Verification items for the finished model (mm, model axes). A direction names the side the tool comes from. Round coordinates to 2 decimals unless told otherwise and drop trailing zeros. Order: outer loops, then holes, each group sorted by start corner. A loop starts at its lowest first (then second) coordinate and runs counter-clockwise, first axis right, second up. Notation, with made-up numbers: M 72,64 L 121,64 A23 ccw 121,93 Z; hole C -34.5,-24 d3. An arc over 180 degrees is marked long. Return JSON: item names as keys, results as strings. Group by question number.
from build123d import *

# Parameters (mm, degrees)
F0_R     = 1
F0_R_2   = 3
F1_DEPTH = 2


with BuildPart() as f1:
    # F0 (on Top) → F1 (new body)
    with BuildSketch(Plane.XY):
        with BuildLine():
            Line((6.85, -35.27), (6.85, -9.66954))
            ThreePointArc((6.85, -9.66954), (10.262401, -5.925), (11.799067, -1.097504))
            Line((11.799067, -1.097504), (33.969716, 11.702726))
            Line((33.969716, 11.702726), (27.119716, 23.567274))
            Line((27.119716, 23.567274), (4.949067, 10.767044))
            ThreePointArc((4.949067, 10.767044), (0, 11.85), (-4.949067, 10.767044))
            Line((-4.949067, 10.767044), (-27.119716, 23.567274))
            Line((-27.119716, 23.567274), (-33.969716, 11.702726))
            Line((-33.969716, 11.702726), (-11.799067, -1.097504))
            ThreePointArc((-11.799067, -1.097504), (-10.262401, -5.925), (-6.85, -9.66954))
            Line((-6.85, -9.66954), (-6.85, -35.27))
            Line((-6.85, -35.27), (6.85, -35.27))
        make_face()
        with Locations((0, -30.4)):
            Circle(F0_R, mode=Mode.SUBTRACT)
        with Locations((0, -16.3)):
            Circle(F0_R, mode=Mode.SUBTRACT)
        with Locations((-6.199088, -5.888446)):
            Circle(F0_R, mode=Mode.SUBTRACT)
        Circle(F0_R_2, mode=Mode.SUBTRACT)
        with Locations((-14.116214, 8.15)):
            Circle(F0_R, mode=Mode.SUBTRACT)
        with Locations((-2, 8.312791)):
            Circle(F0_R, mode=Mode.SUBTRACT)
        with Locations((-26.327172, 15.2)):
            Circle(F0_R, mode=Mode.SUBTRACT)
        with Locations((8.199088, -2.424345)):
            Circle(F0_R, mode=Mode.SUBTRACT)
        with Locations((14.116214, 8.15)):
            Circle(F0_R, mode=Mode.SUBTRACT)
        with Locations((26.327172, 15.2)):
            Circle(F0_R, mode=Mode.SUBTRACT)
    extrude(amount=F1_DEPTH)


solid = f1.part
1. Access from +Z, -Z, +X, -X, +Y, -Y to the whole of each face (thin tool, end or side, straight path). Record for faces 4 (the face through (26.11, 14.224, 0.986)), 5 (the face through (-15.88, 17.08, 0.99)).
2. Thickness scan on line 1 along Y through (x, z) = (0, 0.85); line 2 along X through (y, z) = (-21.5, 1.8); line 3 along X through (y, z) = (-2, 0.9). Record the ranges inside material, lowest first. Write a range as from..to.
3. Cross-section at D-D (y = 0). Enter the section's corners in (x, z).
4. Draft check along X on faces 1 (the face through (0, -35.27, 1)), 2 (the face through (-5.245, -5.588, 0.986)), 3 (the face through (6.85, -23, 1)). Enter one of: +X half, -X half, draft (parallel to the pull), parting line (faces both ways), or undercut.
5. Cross-section at A-A (y = -16.3). Enter the section's corners in (x, z).
6. Cross-section at C-C (z = 0.35). Give the number of separate pieces and of enclosed holes in the cut face, plus the area to 3 significant figures.
7. Cross-section at B-B (x = 0). Enter the section's corners in (y, z).
8. Go/stop test with a flat-tipped pin: pin 1 (0.6 mm diameter, centred on y = -21, z = 1, fed in from +X). Record where the tip stops, or that it passes through.
Computed:
{
 "1": {"face 4": "+Z, -Z", "face 5": "+Z, -Z, +Y"},
 "2": {"line 1": "y = -35.27..-31.4, -29.4..-17.3, -15.3..-3, 3..11.85", "line 2": "x = -6.85..6.85", "line 3": "x = -11.68..-2.24, 2.24..7.29, 9.1..11.68"},
 "3": {"outline": "M -13.7,0 L -3,0 L -3,2 L -13.7,2 Z; M 3,0 L 13.7,0 L 13.7,2 L 3,2 Z"},
 "4": {"face 1": "draft", "face 2": "undercut", "face 3": "+X half"},
 "5": {"outline": "M -6.85,0 L -1,0 L -1,2 L -6.85,2 Z; M 1,0 L 6.85,0 L 6.85,2 L 1,2 Z"},
 "6": {"separate pieces": "1", "enclosed holes": "10", "area": "1,380 mm²"},
 "7": {"outline": "M -35.27,0 L -31.4,0 L -31.4,2 L -35.27,2 Z; M -29.4,0 L -17.3,0 L -17.3,2 L -29.4,2 Z; M -15.3,0 L -3,0 L -3,2 L -15.3,2 Z; M 3,0 L 11.85,0 L 11.85,2 L 3,2 Z"},
 "8": {"pin 1": "stops at x = 6.85"}
}
